Here's how the part is built. I have some questions about the finished solid (model axes, mm). A direction names the side the tool comes from. Round coordinates to 2 decimals unless told otherwise and drop trailing zeros. Order: outer loops, then holes, each group sorted by start corner. A loop starts at its lowest first (then second) coordinate and runs counter-clockwise, first axis right, second up.
```python
from build123d import *

# Parameters (mm, degrees)
BLANKSKE_W          = 200
BLANKSKE_H          = 22.5
BLANK_DEPTH         = 12
TOOTHCUTSIM_DEPTH   = 202.619071519
TEETHCUTS_COUNT     = 26
TEETHCUTS_PITCH     = 7.853981625
SKETCH2_W           = 10
SKETCH2_H           = 90
BOSS_EXTRUDE1_DEPTH = 75
SKETCH3_W           = 200
SKETCH3_H           = 10
BOSS_EXTRUDE2_DEPTH = 10


with BuildPart() as part:
    # BlankSke → Blank (new body)
    with BuildSketch(Plane.XY):
        with Locations((100, 11.25)):
            Rectangle(BLANKSKE_W, BLANKSKE_H)
    extrude(amount=-BLANK_DEPTH)

    # TooCutSkeSim → ToothCutSim (cut, through all)
    with BuildSketch(Plane.XY):
        Polygon((1.087088424, 16.875), (-1.087088424, 16.875), (-3.143665836, 22.5254), (3.143665836, 22.5254), align=None)
    toothcutsim = extrude(amount=-TOOTHCUTSIM_DEPTH, mode=Mode.SUBTRACT)

    # TeethCuts: ToothCutSim ×26
    with Locations(*[(i * TEETHCUTS_PITCH, 0, 0) for i in range(1, TEETHCUTS_COUNT)]):
        add(toothcutsim, mode=Mode.SUBTRACT)

    # Sketch2 → Boss-Extrude1 (add)
    with BuildSketch(Plane.XY):
        with Locations((5, 45)):
            Rectangle(SKETCH2_W, SKETCH2_H)
    extrude(amount=BOSS_EXTRUDE1_DEPTH)

    # Sketch3 → Boss-Extrude2 (add)
    with BuildSketch(Plane(origin=(0, 0, 0), x_dir=(-1, 0, 0), z_dir=(0, 0, -1))):
        with Locations((-100, 85)):
            Rectangle(SKETCH3_W, SKETCH3_H)
    extrude(amount=BOSS_EXTRUDE2_DEPTH)


solid = part.part
```
1. On a 3-axis mill with a long thin cutter (end or side, diameter ignored), from which of +Z, -Z, +X, -X, +Y, -Y can I reach the whole of each face in a straight line? I mean faces 5 (the flat face through (135.643, 19.727, -5.916)), 6 (the flat face through (101, 85, -10)), 7 (the flat face through (9.98, 19.73, -5.92)). Say none if no direction works.
Evaluation:
face 5: +Z, -Z
face 6: -Z, +X, -X, +Y
face 7: -Z
2. If we section it at B-B, the plane z = 31: Write out the boundary of the cut face in (x, y).
Evaluation:
outline: (0, 0) - (10, 0) - (10, 90) - (0, 90) - close
3. If we section it at A-A, the plane y = 48: Write out the boundary of the cut face in (x, z), and give its area (3 significant figures).
Evaluation:
outline: (0, 0) - (10, 0) - (10, 75) - (0, 75) - close
area: 750 mm2
4. I'm going to push a flat-ended pin straight in: P1, Ø3, axis at y = 39.5, z = 12, coming from the +X side. Where does the tip first touch, or does it pass through?
Evaluation:
P1: stops at x = 10
5. I need wall thicknesses on probe 1 along X at (y, z) = (79, 63); probe 2 along Z at (x, y) = (146, 6.5); probe 3 along Z at (x, y) = (136.5, 85). Which ranges of each line are inside material? Lowest first, please.
Evaluation:
probe 1: x = 0 to 10
probe 2: z = -12 to 0
probe 3: z = -10 to 0
6. If we mould it in two halves opening along Y, with no side actions, what happens to faces 1 (the flat face through (21.466, 19.648, -5.916)), 2 (the flat face through (64.96, 19.73, -5.92)), 3 (the flat face through (85, 0, -1)), 4 (the flat face through (78, 90, -2))? For each: released by +Y, released by -Y, zero draft, split by the parting line, or undercut.
Evaluation:
face 1: undercut
face 2: undercut
face 3: released by -Y
face 4: released by +Y
